Study the drawing (mm; zero at the part's minimum x, y, z) and answer. A direction names the side the tool comes from. Give positions to 0.01 mm unless a question says otherwise; leave off trailing zeros. Write each loop counter-clockwise with the first axis right and the second up, starting at its lowest first coordinate (ties: lowest second). Pieces come first, ordered by that corner, then holes. Notation, with made-up numbers: M 17,-4.5 L 61,-4.5 A28 ccw 61,30.5 Z; hole C 84.25,62.25 d4. An arc over 180 degrees is marked long. Use a Markdown table: item, result. Add a question column.
Item 1: Consider probe 1 along X at (y, z) = (1.25, 7); probe 2 along Z at (x, y) = (24, 3) (1 decimal); probe 3 along Z at (x, y) = (7.5, 9) (1 decimal). Determine where each line is inside the solid, lowest interval first. Write a range as [from, to].
Item 2: For the marked faces 1, 2, 3 and 4, determine the directions among +Z, -Z, +X, -X, +Y, -Y from which every point of the face is accessible in a straight line to the end or side of a thin tool.
Item 3: A cutting plane is placed at B-B on x = 4. Determine the outline of the cut face in (y, z) (1 decimal).
Item 4: A cutting plane is placed at A-A on y = 5. Count the separate pieces of the cut face and the enclosed holes in it.
Item 5: Given P1, Ø6, axis at x = 4.5, z = 8.5, coming from the -Y side; P2, Ø5, axis at y = 7, z = 6, coming from the +X side; P3, Ø6, axis at x = 24, y = 8.5, coming from the +Z side, each flat-ended and moving along its own axis, determine where each tip first touches the part or whether it passes through.
Item 6: A cutting plane is placed at D-D on z = 24.5. Determine the outline of the cut face in (x, y).
Item 7: The mould has two halves that part along Z. Classify the marked faces 5, 6, 7 and 8: pulls with the +Z half, pulls with the -Z half, needs draft (parallel to the pull), parting line crosses it, or undercut.
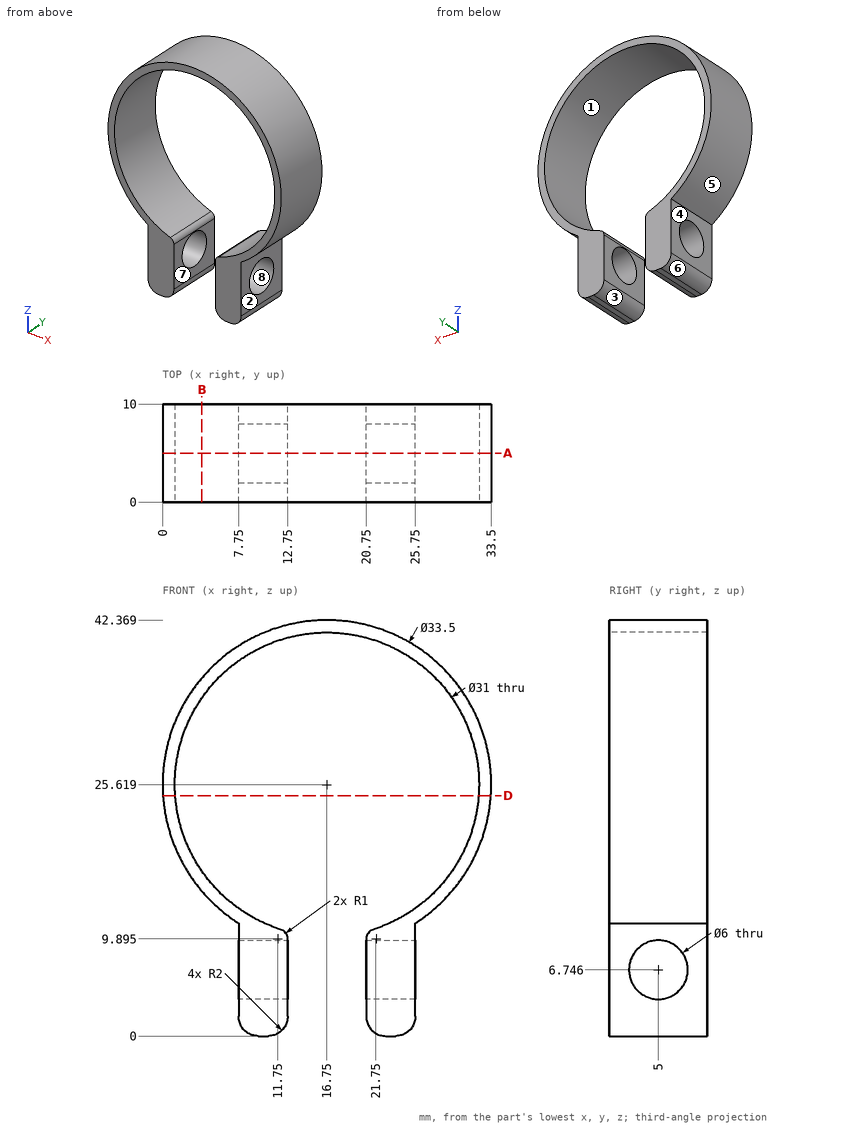
Filled in:
| question | item | result |
|---|---|---|
| 1 | probe 1 | [7.75, 12.75], [20.75, 25.75] |
| 1 | probe 2 | [0, 4.5], [9, 11.9], [39.3, 40.7] |
| 1 | probe 3 | [11.7, 13.2], [38.1, 39.6] |
| 2 | face 1 | +Y, -Y |
| 2 | face 2 | -Z, +X, +Y, -Y |
| 2 | face 3 | -Z, +Y, -Y |
| 2 | face 4 | -Z, -X, +Y, -Y |
| 3 | outline | M 0,14.8 L 10,14.8 L 10,16.8 L 0,16.8 Z; M 0,34.4 L 10,34.4 L 10,36.5 L 0,36.5 Z |
| 4 | separate pieces | 3 |
| 4 | enclosed holes | 0 |
| 5 | P1 | through |
| 5 | P2 | x = 25.75 |
| 5 | P3 | z = 41.82 |
| 6 | outline | M 0.04,0 L 1.29,0 L 1.29,10 L 0.04,10 Z; M 32.21,0 L 33.46,0 L 33.46,10 L 32.21,10 Z |
| 7 | face 5 | parting line crosses it |
| 7 | face 6 | pulls with the -Z half |
| 7 | face 7 | needs draft |
| 7 | face 8 | undercut |
